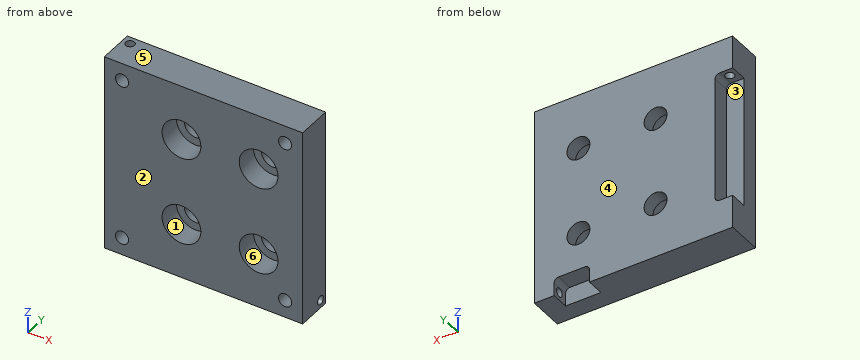
from build123d import *

# Parameters (mm, degrees)
SKETCH_1_W           = 45
SKETCH_1_H           = 45
EXTRUDE_1_DEPTH      = 8
SKETCH_2_R           = 2.6
CUT_EXTRUDE_1_DEPTH  = 9
SKETCH_3_R           = 4.4
CUT_EXTRUDE_2_DEPTH  = 5
SKETCH_5_W           = 4
SKETCH_5_H           = 30
CUT_EXTRUDE_4_DEPTH  = 4
SKETCH_6_R           = 1
CUT_EXTRUDE_5_DEPTH  = 9
FILLET_1_R           = 1
SKETCH_7_W           = 8
SKETCH_7_H           = 4
CUT_EXTRUDE_6_DEPTH  = 4
FILLET_2_R           = 1
SKETCH_8_R           = 1
CUT_EXTRUDE_7_DEPTH  = 9
SKETCH_11_R          = 1.5
CUT_EXTRUDE_10_DEPTH = 3


with BuildPart() as part:
    # 草图1 → 凸台-拉伸1 (new body)
    with BuildSketch(Plane(origin=(0, 0, 0), x_dir=(1, 0, 0), z_dir=(0, 1, 0))):
        with Locations((22.5, 22.5)):
            Rectangle(SKETCH_1_W, SKETCH_1_H)
    extrude(amount=EXTRUDE_1_DEPTH)

    # 草图2 → 切除-拉伸1 (cut, through all)
    with BuildSketch(Plane(origin=(0, 8, 0), x_dir=(1, 0, 0), z_dir=(0, 1, 0))):
        with Locations((17.5, 12.5)):
            Circle(SKETCH_2_R)
        with Locations((17.5, 32.5)):
            Circle(SKETCH_2_R)
        with Locations((35, 12.5)):
            Circle(SKETCH_2_R)
        with Locations((35, 32.5)):
            Circle(SKETCH_2_R)
    extrude(amount=-CUT_EXTRUDE_1_DEPTH, mode=Mode.SUBTRACT)

    # 草图3 → 切除-拉伸2 (cut)
    with BuildSketch(Plane(origin=(0, 0, 0), x_dir=(-1, 0, 0), z_dir=(0, -1, 0))):
        with Locations((-17.5, 32.5)):
            Circle(SKETCH_3_R)
        with Locations((-17.5, 12.5)):
            Circle(SKETCH_3_R)
        with Locations((-35, 12.5)):
            Circle(SKETCH_3_R)
        with Locations((-35, 32.5)):
            Circle(SKETCH_3_R)
    extrude(amount=-CUT_EXTRUDE_2_DEPTH, mode=Mode.SUBTRACT)

    # 草图5 → 切除-拉伸4 (cut)
    with BuildSketch(Plane(origin=(0, 8, 0), x_dir=(1, 0, 0), z_dir=(0, 1, 0))):
        with Locations((2, 22.5)):
            Rectangle(SKETCH_5_W, SKETCH_5_H)
    extrude(amount=-CUT_EXTRUDE_4_DEPTH, mode=Mode.SUBTRACT)

    # 草图6 → 切除-拉伸5 (cut)
    with BuildSketch(Plane.XY):
        with Locations((1.8, 6.2)):
            Circle(SKETCH_6_R)
    extrude(amount=-CUT_EXTRUDE_5_DEPTH, mode=Mode.SUBTRACT)

    # 圆角1
    fillet_1_edges = [part.edges().sort_by_distance(p)[0] for p in [
        (4, 6, -37.5),
        (4, 6, -7.5),
    ]]
    fillet(fillet_1_edges, radius=FILLET_1_R)

    # 草图7 → 切除-拉伸6 (cut)
    with BuildSketch(Plane(origin=(0, 8, 0), x_dir=(1, 0, 0), z_dir=(0, 1, 0))):
        with Locations((36.5, 43)):
            Rectangle(SKETCH_7_W, SKETCH_7_H)
    extrude(amount=-CUT_EXTRUDE_6_DEPTH, mode=Mode.SUBTRACT)

    # 圆角2
    fillet_2_edges = [part.edges().sort_by_distance(p)[0] for p in [
        (40.5, 6, -41),
        (32.5, 6, -41),
    ]]
    fillet(fillet_2_edges, radius=FILLET_2_R)

    # 草图8 → 切除-拉伸7 (cut)
    with BuildSketch(Plane(origin=(45, 0, 0), x_dir=(0, 0, -1), z_dir=(1, 0, 0))):
        with Locations((43.2, 6.2)):
            Circle(SKETCH_8_R)
    extrude(amount=-CUT_EXTRUDE_7_DEPTH, mode=Mode.SUBTRACT)

    # 草图11 → 切除-拉伸10 (cut)
    with BuildSketch(Plane(origin=(0, 0, 0), x_dir=(-1, 0, 0), z_dir=(0, -1, 0))):
        with Locations((-4, 4)):
            Circle(SKETCH_11_R)
        with Locations((-41, 4)):
            Circle(SKETCH_11_R)
        with Locations((-4, 41)):
            Circle(SKETCH_11_R)
        with Locations((-41, 41)):
            Circle(SKETCH_11_R)
    extrude(amount=-CUT_EXTRUDE_10_DEPTH, mode=Mode.SUBTRACT)


solid = part.part
Could you check a few things on this model? Use its own coordinates, in mm. Face numbers are marked on the shaded views. A direction names the side the tool comes from. Give positions to 0.01 mm unless a question says otherwise; leave off trailing zeros. Write each loop counter-clockwise with the first axis right and the second up, starting at its lowest first coordinate (ties: lowest second). Pieces come first, ordered by that corner, then holes. Notation, with made-up numbers: (11.5, 14) -> (58.5, 14) arc R21 cw to (58.5, 45) -> close; hole circle Ø4 at (-7, 62.25). An arc over 180 degrees is marked (long way). Answer as CSV lines item,"result". Start each with the question number.
(1) If we mould it in two halves opening along Z, with no side actions, what happens to the marked faces 4, 5 and 6? For each: +Z half, -Z half, draft (parallel to the pull), parting line (faces both ways), or undercut.
(2) If we section it at C-C, the plane y = 2.25: Give the number of separate pieces and of enclosed holes in the cut face, and give its area (3 significant figures).
(3) If we section it at B-B, the plane z = -4: Write out the boundary of the cut face in (x, y).
(4) Which directions (+Z, -Z, +X, -X, +Y, -Y) give clear straight access to the entire face, cutting with the end or side of a thin tool? Please do the marked faces 1, 2 and 3.
(5) If we section it at A-A, the plane x = 17.5: Write out the boundary of the cut face in (y, z), and give its area (3 significant figures).
(6) I'm going to push flat-ended pins straight in: pin 1 Ø2.5 at (x, z) = (18.5, -10.5) entering from -Y; pin 2 Ø0.9 at (x, z) = (41, -41.5) entering from -Y; pin 3 Ø2 at (x, z) = (1.5, -26) entering from +Y. Where does each tip first touch, or does it pass through?
(7) If we section it at D-D, the plane x = 41.5: Write out the boundary of the cut face in (y, z).
(8) Please list where these lines run through material, in increasing order: line 1 (Z direction, x = 17.5, y = 6.2); line 2 (Z direction, x = 35, y = 2.45); line 3 (X direction, y = 3.75, z = -32.5).
Answer list:
1,face 4,"draft"
1,face 5,"+Z half"
1,face 6,"undercut"
2,separate pieces,"1"
2,enclosed holes,"8"
2,area,"1,750 mm^2"
3,outline,"(0, 0) -> (2.5, 0) -> (2.5, 3) -> (5.5, 3) -> (5.5, 0) -> (39.5, 0) -> (39.5, 3) -> (42.5, 3) -> (42.5, 0) -> (45, 0) -> (45, 8) -> (0, 8) -> close; hole circle Ø2 at (1.8, 6.2)"
4,face 1,"-Y"
4,face 2,"+Z, -Z, +X, -X, -Y"
4,face 3,"-X, +Y"
5,outline,"(0, -45) -> (8, -45) -> (8, -35.1) -> (5, -35.1) -> (5, -36.9) -> (0, -36.9) -> close; (0, -28.1) -> (5, -28.1) -> (5, -29.9) -> (8, -29.9) -> (8, -15.1) -> (5, -15.1) -> (5, -16.9) -> (0, -16.9) -> close; (0, -8.1) -> (5, -8.1) -> (5, -9.9) -> (8, -9.9) -> (8, 0) -> (0, 0) -> close"
5,area,"241 mm^2"
6,pin 1,"y = 5"
6,pin 2,"y = 3"
6,pin 3,"y = 4"
7,outline,"(0, -45) -> (8, -45) -> (8, 0) -> (0, 0) -> (0, -2.59) -> (3, -2.59) -> (3, -5.41) -> (0, -5.41) -> (0, -39.59) -> (3, -39.59) -> (3, -42.41) -> (0, -42.41) -> close; hole circle Ø2 at (6.2, -43.2)"
8,line 1,"-45 to -35.1, -29.9 to -15.1, -9.9 to 0"
8,line 2,"-45 to -36.9, -28.1 to -16.9, -8.1 to 0"
8,line 3,"0 to 13.1, 21.9 to 30.6, 39.4 to 45"
